from build123d import *

# Parameters (mm, degrees)
SKETCH1_W                = 133.7
SKETCH1_H                = 96.52
BOSS_EXTRUDE2_DEPTH      = 3
SKETCH6_W                = 48.26
SKETCH6_H                = 3
CUT_EXTRUDE2_DEPTH       = 3
SKETCH9_W                = 16.086666666
SKETCH9_H                = 3
BOSS_EXTRUDE4_DEPTH      = 3
SKETCH11_W               = 31.925
SKETCH11_H               = 3
CUT_EXTRUDE8_DEPTH       = 3
SKETCH15_W               = 10.641666666
SKETCH15_H               = 3
BOSS_EXTRUDE7_DEPTH      = 3
SKETCH18_W               = 31.925
SKETCH18_H               = 3
CUT_EXTRUDE10_DEPTH      = 3
SKETCH19_W               = 10.64166667
SKETCH19_H               = 3
BOSS_EXTRUDE8_DEPTH      = 3
SKETCH21_R               = 1.45
CUT_EXTRUDE11_DEPTH      = 3
MIRROR16_COPY_1_SKETCH_R = 1.45
MIRROR16_COPY_1_DEPTH    = 3
SKETCH22_R               = 1.45
CUT_EXTRUDE19_DEPTH      = 3
SKETCH24_R               = 1.6
CUT_EXTRUDE20_DEPTH      = 3
SKETCH25_W               = 15
SKETCH25_H               = 3
CUT_EXTRUDE21_DEPTH      = 3


with BuildPart() as part:
    # Sketch1 → Boss-Extrude2 (new body)
    with BuildSketch(Plane(origin=(0, 0, 0), x_dir=(1, 0, 0), z_dir=(0, 1, 0))):
        Rectangle(SKETCH1_W, SKETCH1_H)
    extrude(amount=BOSS_EXTRUDE2_DEPTH)

    # Sketch6 → Cut-Extrude2 (cut)
    with BuildSketch(Plane.ZY.offset(66.85)):
        with Locations((0, 1.5)):
            Rectangle(SKETCH6_W, SKETCH6_H)
    cut_extrude2 = extrude(amount=-CUT_EXTRUDE2_DEPTH, mode=Mode.SUBTRACT)

    # Mirror3: Cut-Extrude2 across plane
    add(cut_extrude2.mirror(Plane(origin=(0, 0, 0), x_dir=(0, 0, 1), z_dir=(1, 0, 0))), mode=Mode.SUBTRACT)

    # Sketch9 → Boss-Extrude4 (add)
    with BuildSketch(Plane(origin=(63.85, 0, 0), x_dir=(0, 0, -1), z_dir=(1, 0, 0))):
        with Locations((0, 1.5)):
            Rectangle(SKETCH9_W, SKETCH9_H)
    boss_extrude4 = extrude(amount=BOSS_EXTRUDE4_DEPTH)

    # Mirror5: Boss-Extrude4 across plane
    add(boss_extrude4.mirror(Plane(origin=(0, 0, 0), x_dir=(0, 0, 1), z_dir=(1, 0, 0))))

    # Sketch11 → Cut-Extrude8 (cut)
    with BuildSketch(Plane.XY.offset(48.26)):
        with Locations((-33.425, 1.5)):
            Rectangle(SKETCH11_W, SKETCH11_H)
    cut_extrude8 = extrude(amount=-CUT_EXTRUDE8_DEPTH, mode=Mode.SUBTRACT)

    # Sketch15 → Boss-Extrude7 (add)
    with BuildSketch(Plane.XY.offset(45.26)):
        with Locations((-33.425, 1.5)):
            Rectangle(SKETCH15_W, SKETCH15_H)
    boss_extrude7 = extrude(amount=BOSS_EXTRUDE7_DEPTH)

    # Mirror11: Cut-Extrude8 across plane
    add(cut_extrude8.mirror(Plane.XY), mode=Mode.SUBTRACT)

    # Mirror12: Boss-Extrude7 across plane
    add(boss_extrude7.mirror(Plane.XY))

    # Sketch18 → Cut-Extrude10 (cut)
    with BuildSketch(Plane.XY.offset(48.26)):
        with Locations((33.425, 1.5)):
            Rectangle(SKETCH18_W, SKETCH18_H)
    cut_extrude10 = extrude(amount=-CUT_EXTRUDE10_DEPTH, mode=Mode.SUBTRACT)

    # Sketch19 → Boss-Extrude8 (add)
    with BuildSketch(Plane.XY.offset(45.26)):
        with Locations((33.425, 1.5)):
            Rectangle(SKETCH19_W, SKETCH19_H)
    boss_extrude8 = extrude(amount=BOSS_EXTRUDE8_DEPTH)

    # Mirror13: Cut-Extrude10 across plane
    add(cut_extrude10.mirror(Plane.XY), mode=Mode.SUBTRACT)

    # Mirror14: Boss-Extrude8 across plane
    add(boss_extrude8.mirror(Plane.XY))

    # Sketch21 → Cut-Extrude11 (cut)
    with BuildSketch(Plane(origin=(0, 3, 0), x_dir=(1, 0, 0), z_dir=(0, 1, 0))):
        with Locations((33.375833335, -46.91)):
            Circle(SKETCH21_R)
    cut_extrude11 = extrude(amount=-CUT_EXTRUDE11_DEPTH, mode=Mode.SUBTRACT)

    # Mirror15: Cut-Extrude11 across plane
    add(cut_extrude11.mirror(Plane.XY), mode=Mode.SUBTRACT)

    # Mirror16: Cut-Extrude11 across plane
    add(cut_extrude11.mirror(Plane(origin=(0, 0, 0), x_dir=(0, 0, 1), z_dir=(1, 0, 0))), mode=Mode.SUBTRACT)

    # Mirror16 copy 1 sketch → Mirror16 copy 1 (cut)
    with BuildSketch(Plane(origin=(0, 3, 0), x_dir=(-1, 0, 0), z_dir=(0, 1, 0))):
        with Locations((33.375833335, -46.91)):
            Circle(MIRROR16_COPY_1_SKETCH_R)
    extrude(amount=-MIRROR16_COPY_1_DEPTH, mode=Mode.SUBTRACT)

    # Sketch22 → Cut-Extrude19 (cut)
    with BuildSketch(Plane(origin=(0, 3, 0), x_dir=(1, 0, 0), z_dir=(0, 1, 0))):
        with Locations((65.5, 0)):
            Circle(SKETCH22_R)
    cut_extrude19 = extrude(amount=-CUT_EXTRUDE19_DEPTH, mode=Mode.SUBTRACT)

    # Mirror17: Cut-Extrude19 across plane
    add(cut_extrude19.mirror(Plane(origin=(0, 0, 0), x_dir=(0, 0, 1), z_dir=(1, 0, 0))), mode=Mode.SUBTRACT)

    # Sketch24 → Cut-Extrude20 (cut)
    with BuildSketch(Plane(origin=(0, 3, 0), x_dir=(1, 0, 0), z_dir=(0, 1, 0))):
        with Locations((-53.75, -40.14)):
            Circle(SKETCH24_R)
        with Locations((-25.85, -40.14)):
            Circle(SKETCH24_R)
        with Locations((-10.55, 10.66)):
            Circle(SKETCH24_R)
        with Locations((-58.85, 12.26)):
            Circle(SKETCH24_R)
    extrude(amount=-CUT_EXTRUDE20_DEPTH, mode=Mode.SUBTRACT)

    # Sketch25 → Cut-Extrude21 (cut)
    with BuildSketch(Plane(origin=(0, 3, 0), x_dir=(1, 0, 0), z_dir=(0, 1, 0))):
        with Locations((4.75, 16.76)):
            Rectangle(SKETCH25_W, SKETCH25_H)
    extrude(amount=-CUT_EXTRUDE21_DEPTH, mode=Mode.SUBTRACT)


solid = part.part
Source: CAD feature listing. Evaluate the final solid. Frame: model axes, mm. A direction names the side the tool comes from. Coordinates: 2 decimals unless noted, no trailing zeros. Write each loop counter-clockwise with the first axis right and the second up, starting at its lowest first coordinate (ties: lowest second). Pieces come first, ordered by that corner, then holes. Notation, with made-up numbers: M 26,-24 L 60,-24 A33 cw 60,12 Z; hole C 37,7 d3. An arc over 180 degrees is marked long. Use a Markdown table: item, result.
1) Section A-A, the plane z = 40.14. Output: boundary loops of the cut face in (x, y).
Conclusion:
| item | result |
|---|---|
| outline | M -66.85,0 L -55.35,0 L -55.35,3 L -66.85,3 Z; M -52.15,0 L -27.45,0 L -27.45,3 L -52.15,3 Z; M -24.25,0 L 66.85,0 L 66.85,3 L -24.25,3 Z |
2) Section D-D, the plane y = 2.1. Give the number of separate pieces and of enclosed holes in the cut face, then the cut area to 3 significant figures.
Conclusion:
| item | result |
|---|---|
| separate pieces | 1 |
| enclosed holes | 5 |
| area | 12,300 mm^2 |
3) Ray query, L1, parallel to Z at x = -10.55, y = 1.4; L2, parallel to X at y = 0.9, z = -18; L3, parallel to X at y = 2.75, z = 41. Return the intervals inside material, ascending.
Conclusion:
| item | result |
|---|---|
| L1 | z = -48.26 to -12.26, -9.06 to 48.26 |
| L2 | x = -63.85 to -2.75, 12.25 to 63.85 |
| L3 | x = -66.85 to -55.1, -52.4 to -27.2, -24.5 to 66.85 |
4) First-contact query: pin 1 Ø2.5 at (x, z) = (-65.5, 0) entering from -Y; pin 2 Ø1.5 at (x, y) = (-21.5, 1) entering from -Z. Flat tips, straight axial feed; report the tip coordinate or a pass-through.
Conclusion:
| item | result |
|---|---|
| pin 1 | passes through |
| pin 2 | stops at z = -45.26 |
5) Section B-B, the plane x = -58.85. Output: boundary loops of the cut face in (y, z).
Conclusion:
| item | result |
|---|---|
| outline | M 0,-48.26 L 3,-48.26 L 3,-13.86 L 0,-13.86 Z; M 0,-10.66 L 3,-10.66 L 3,48.26 L 0,48.26 Z |
6) Mould query, pull axis X, two halves, no side actions, for faces 1 (the flat face through (-23, 2, 45.26)), 2 (the flat face through (66.85, 1, -36)), 3 (the flat face through (-1, 0, -1)). Classes: pulls with the +X half, pulls with the -X half, needs draft (parallel to the pull), parting line crosses it, or undercut.
Conclusion:
| item | result |
|---|---|
| face 1 | undercut |
| face 2 | pulls with the +X half |
| face 3 | needs draft |
7) Section C-C, the plane z = -46.91. Output: boundary loops of the cut face in (x, y), then the cut area to 3 significant figures.
Conclusion:
| item | result |
|---|---|
| outline | M -66.85,0 L -49.39,0 L -49.39,3 L -66.85,3 Z; M -38.75,0 L -34.83,0 L -34.83,3 L -38.75,3 Z; M -31.93,0 L -28.1,0 L -28.1,3 L -31.93,3 Z; M -17.46,0 L 17.46,0 L 17.46,3 L -17.46,3 Z; M 28.1,0 L 31.93,0 L 31.93,3 L 28.1,3 Z; M 34.83,0 L 38.75,0 L 38.75,3 L 34.83,3 Z; M 49.39,0 L 66.85,0 L 66.85,3 L 49.39,3 Z |
| area | 256 mm^2 |
8) Reachability of faces 4 (the flat face through (63.85, 2, 16)), 5 (the flat face through (5, 2, -18.26)), 6 (the flat face through (28.104, 1, -47)) from +Z, -Z, +X, -X, +Y, -Y: full face, straight path, thin tool, end or side. Return the list, or none.
Conclusion:
| item | result |
|---|---|
| face 4 | +X, +Y, -Y |
| face 5 | +Y, -Y |
| face 6 | -Z, +Y, -Y |
